```python
from build123d import *

# Parameters (mm, degrees)
SKETCH1_W           = 490
SKETCH1_H           = 300
BOSS_EXTRUDE1_DEPTH = 18
SKETCH5_W           = 9
SKETCH5_H           = 300
CUT_EXTRUDE1_DEPTH  = 18
SKETCH6_W           = 18
SKETCH6_H           = 300
CUT_EXTRUDE3_DEPTH  = 9


with BuildPart() as part:
    # Sketch1 → Boss-Extrude1 (new body)
    with BuildSketch(Plane(origin=(0, 0, 0), x_dir=(0, 0, -1), z_dir=(1, 0, 0))):
        with Locations((245, 150)):
            Rectangle(SKETCH1_W, SKETCH1_H)
    extrude(amount=BOSS_EXTRUDE1_DEPTH)

    # Sketch5 → Cut-Extrude1 (cut)
    with BuildSketch(Plane.XY):
        with Locations((4.5, 150)):
            Rectangle(SKETCH5_W, SKETCH5_H)
    extrude(amount=-CUT_EXTRUDE1_DEPTH, mode=Mode.SUBTRACT)

    # Sketch6 → Cut-Extrude3 (cut)
    with BuildSketch(Plane.ZY):
        with Locations((-481, 150)):
            Rectangle(SKETCH6_W, SKETCH6_H)
    extrude(amount=-CUT_EXTRUDE3_DEPTH, mode=Mode.SUBTRACT)


solid = part.part
```
Design review of the part built by this model. Coordinates are the model's own, in mm. A direction names the side the tool comes from. Give positions to 0.01 mm unless a question says otherwise; leave off trailing zeros. Write each loop counter-clockwise with the first axis right and the second up, starting at its lowest first coordinate (ties: lowest second). Pieces come first, ordered by that corner, then holes. Notation, with made-up numbers: (50, 37) -> (107, 37) arc R9 ccw to (107, 54) -> close; hole circle Ø9 at (-39.5, 0). An arc over 180 degrees is marked (long way). Answer in a Markdown table with one row per item.
(1) Consider section A-A (y = 155). State the section outline as (x, z) points.
Results:
| item | result |
|---|---|
| outline | (0, -472) -> (9, -472) -> (9, -490) -> (18, -490) -> (18, 0) -> (9, 0) -> (9, -18) -> (0, -18) -> close |
(2) Consider section B-B (x = 6). State the section outline as (y, z) points, then the cut area to 3 significant figures.
Results:
| item | result |
|---|---|
| outline | (0, -472) -> (300, -472) -> (300, -18) -> (0, -18) -> close |
| area | 136,000 mm2 |
(3) To check wall thickness, follow probe 1 along Z at (x, y) = (3.75, 219). State the ranges of the line that lie inside material, in increasing order.
Results:
| item | result |
|---|---|
| probe 1 | -472 to -18 |
(4) Clearance check with flat-ended pins moving along their axes: pin 1 (6 mm diameter, centred on x = 3.5, y = 103.5, fed in from -Z); pin 2 (5.5 mm diameter, centred on y = 177, z = -479, fed in from -X); pin 3 (4.5 mm diameter, centred on x = 5, y = 216.5, fed in from +Z). State where each tip first meets the part, or that it passes through.
Results:
| item | result |
|---|---|
| pin 1 | z = -472 |
| pin 2 | x = 9 |
| pin 3 | z = -18 |
(5) For faces 1 (the flat face through (4, 152, -18)), 2 (the flat face through (9, 152, -481)), 3 (the flat face through (0, 152, -242)), list the 3-axis set-ups (+Z, -Z, +X, -X, +Y, -Y) from which the entire face can be reached by the end or side of a thin tool; tool diameter is ignored.
Results:
| item | result |
|---|---|
| face 1 | +Z, -X, +Y, -Y |
| face 2 | -Z, -X, +Y, -Y |
| face 3 | +Z, -Z, -X, +Y, -Y |
